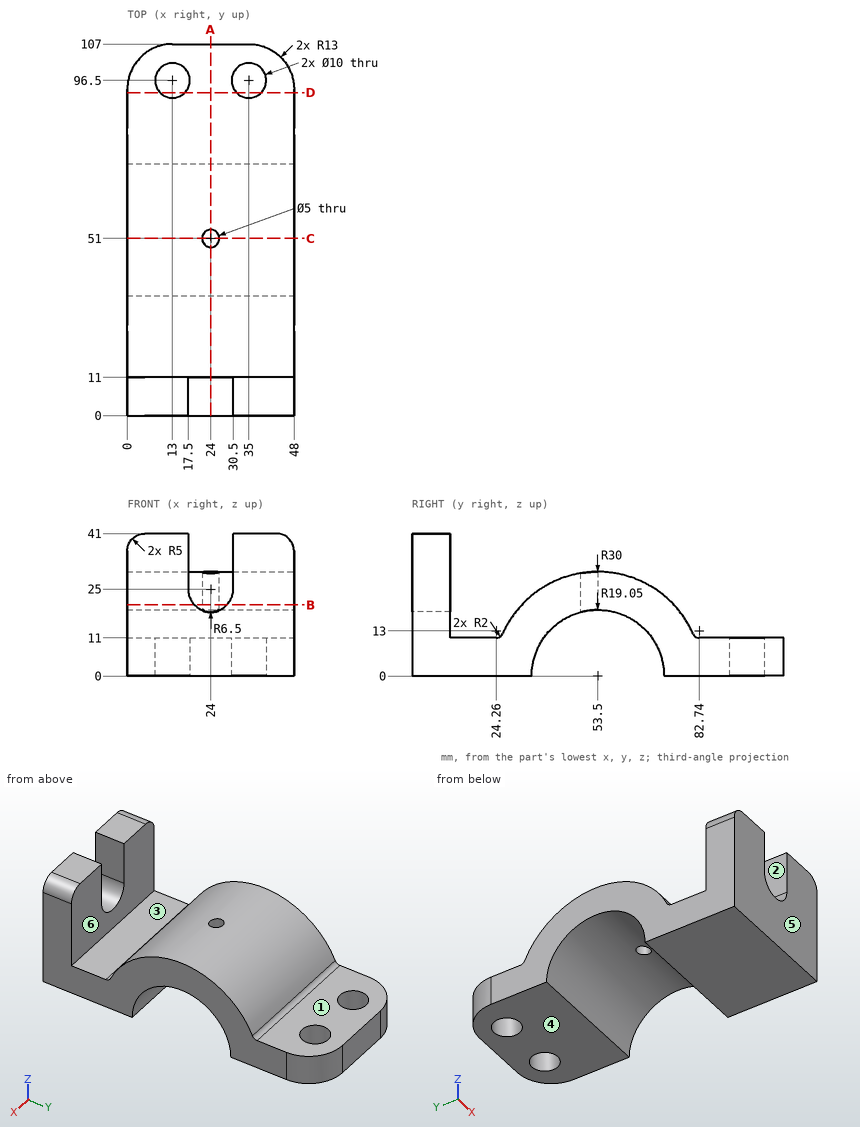
Answer from the drawing. Dimensions are ordinates in mm from the lowest x, y and z of the part. A direction names the side the tool comes from. Coordinates: 2 decimals unless noted, no trailing zeros. Write each loop counter-clockwise with the first axis right and the second up, starting at its lowest first coordinate (ties: lowest second). Pieces come first, ordered by that corner, then holes. Notation, with made-up numbers: (4.25, 30) - (44.25, 30) arc R31 ccw to (44.25, 67) - close; hole circle Ø9 at (40, -34). An arc over 180 degrees is marked (long way). Return JSON: item names as keys, results as strings. Group by question number.
Q1. Find the intervals of material crossed by line 1 along Y through (x, z) = (36.5, 17) (1 decimal); line 2 along X through (y, z) = (96, 7) (1 decimal); line 3 along X through (y, z) = (51, 22.75), in increasing order. Write a range as [from, to].
Q2. The part is cut by section B-B on z = 20.5. Write down the section's boundary in (x, y), and give its area (3 significant figures).
Q3. The part is cut by section D-D on y = 93. Write down the section's boundary in (x, z).
Q4. Which of the six approach directions +Z, -Z, +X, -X, +Y, -Y give full straight-line access (tool end or side, diameter ignored) to the marked faces 1, 2 and 3?
Q5. For a pull along Y with two mould halves and no side action, classify the marked faces 4, 5 and 6 as +Y half, -Y half, draft (parallel to the pull), parting line (faces both ways), or undercut.
Q6. Flat-ended cylindrical pins translate along their axes: pin 1 Ø12 at (x, y) = (12.5, 72.5) entering from +Z; pin 2 Ø10.5 at (x, y) = (23.5, 16) entering from +Z; pin 3 Ø2 at (x, z) = (31.5, 36) entering from +Y; pin 4 Ø8 at (x, y) = (35, 96.5) entering from -Z. Find the tip coordinate at first contact, or state that the pin passes through.
Q7. The part is cut by section A-A on x = 24. Write down the section's boundary in (y, z).
Q8. The part is cut by section C-C on y = 51. Write down the section's boundary in (x, z) (1 decimal).
Evaluation:
{
 "1": {"line 1": "y = [0, 11], [28.8, 44.9], [62.1, 78.2]", "line 2": "x = [0.2, 8], [18, 30], [40, 47.8]", "line 3": "x = [0, 21.5], [26.5, 48]"},
 "2": {"outline": "(0, 0) - (19.31, 0) - (19.31, 11) - (0, 11) - close; (0, 31.6) - (48, 31.6) - (48, 75.4) - (0, 75.4) - close; (28.69, 0) - (48, 0) - (48, 11) - (28.69, 11) - close; hole circle Ø5 at (24, 51)", "area": "2,510 mm2"},
 "3": {"outline": "(0, 0) - (9.43, 0) - (9.43, 11) - (0, 11) - close; (16.57, 0) - (31.43, 0) - (31.43, 11) - (16.57, 11) - close; (38.57, 0) - (48, 0) - (48, 11) - (38.57, 11) - close"},
 "4": {"face 1": "+Z, +X, -X, +Y", "face 2": "+Z, -Y", "face 3": "+Z, +X, -X"},
 "5": {"face 4": "draft", "face 5": "-Y half", "face 6": "undercut"},
 "6": {"pin 1": "stops at z = 27.04", "pin 2": "stops at z = 18.85", "pin 3": "stops at y = 11", "pin 4": "passes through"},
 "7": {"outline": "(0, 0) - (34.45, 0) arc R19.05 cw to (48.5, 18.38) - (48.5, 29.58) arc R30 ccw to (26.09, 12.19) arc R2 cw to (24.26, 11) - (11, 11) - (11, 18.5) - (0, 18.5) - close; (53.5, 19.05) arc R19.05 cw to (72.55, 0) - (107, 0) - (107, 11) - (82.74, 11) arc R2 cw to (80.91, 12.19) arc R30 ccw to (53.5, 30) - close"},
 "8": {"outline": "(0, 18.9) - (21.5, 18.9) - (21.5, 29.9) - (0, 29.9) - close; (26.5, 18.9) - (48, 18.9) - (48, 29.9) - (26.5, 29.9) - close"}
}
